Could you check a few things on this model? Use its own coordinates, in mm. A direction names the side the tool comes from. Give positions to 0.01 mm unless a question says otherwise; leave off trailing zeros. Order: outer loops, then holes, each group sorted by start corner. A loop starts at its lowest first (then second) coordinate and runs counter-clockwise, first axis right, second up. Notation, with made-up numbers: (4, 23) - (61, 23) arc R11 ccw to (61, 44) - close; hole circle Ø4 at (57.5, 18.25). An arc over 180 degrees is marked (long way). One line per question, with ' | ' between items. Start each with the question number.
1. Which directions (+Z, -Z, +X, -X, +Y, -Y) give clear straight access to the entire face, cutting with the end or side of a thin tool? Please do faces 5 (the flat face through (1.8, 0, 18)), 6 (the flat face through (1.8, 0, -18)), 7 (the flat face through (1.8, -13, -13)), 8 (the flat face through (6, -14, 0)).
2. Imagine slicing it at A-A (y = 18.5). Please give me the cut outline in (x, z).
3. If we mould it in two halves opening along Z, with no side actions, what happens to faces 1 (the cylindrical face through (2.96, 7.28, -23.13)), 2 (the flat face through (-79, 27.848, 0)), 3 (the cylindrical face through (3.871, 14.888, 13.165)), 4 (the flat face through (1.8, 13, -13))? For each: released by +Z, released by -Z, zero draft, split by the parting line, or undercut.
4. I need wall thicknesses on probe 1 along X at (y, z) = (-10, 2.5); probe 2 along Z at (x, y) = (-78.5, 22.5); probe 3 along X at (y, z) = (17, 12.5). Which ranges of each line are inside material? Lowest first, please. Write a range as from..to.
5. For P1, Ø5, axis at x = -71, z = -6, coming from the -Y side; P2, Ø20.5, axis at y = 6, z = 1.5, coming from the +X side; P3, Ø8, axis at x = 8.5, z = -10.5, coming from the -Y side; P4, Ø4, axis at x = -31.5, y = -18.5, coming from the -Z side, each with a flat end and sliding along its axis, tell me the tip position at first contact or that it passes through.
6. Imagine slicing it at B-B (x = -20.5). Please give me the cut outline in (y, z), and give its area (3 significant figures).
```python
from build123d import *
from build123d.topology import SkipClean

# Parameters (mm, degrees)
SKETCH1_R           = 24.6
BOSS_EXTRUDE1_DEPTH = 87
SKETCH2_R           = 24.25
BOSS_EXTRUDE2_DEPTH = 6
BOSS_EXTRUDE3_DEPTH = 5
CUT_EXTRUDE1_START  = -4.2
SKETCH4_R           = 5.5
SKETCH4_R_2         = 2
CUT_EXTRUDE1_DEPTH  = 4.2
CUT_EXTRUDE2_START  = -0.5
CUT_EXTRUDE2_DEPTH  = 0.5
SKETCH6_R           = 12.7
SKETCH6_R_2         = 5.5
BOSS_EXTRUDE4_DEPTH = 2.5
SKETCH7_R           = 10
SKETCH7_R_2         = 8.5
CUT_EXTRUDE3_DEPTH  = 0.5
SKETCH8_R           = 4
BOSS_EXTRUDE5_DEPTH = 33
CUT_EXTRUDE4_DEPTH  = 3.5
BOSS_EXTRUDE7_START = 22
BOSS_EXTRUDE7_DEPTH = 22


with BuildPart() as part:
    # Sketch1 → Boss-Extrude1 (new body)
    with BuildSketch(Plane(origin=(0, 0, 0), x_dir=(0, 0, -1), z_dir=(1, 0, 0))):
        Circle(SKETCH1_R)
    extrude(amount=-BOSS_EXTRUDE1_DEPTH)

    # Sketch2 → Boss-Extrude2 (add)
    with BuildSketch(Plane(origin=(0, 0, 0), x_dir=(0, 0, -1), z_dir=(1, 0, 0))):
        Circle(SKETCH2_R)
    extrude(amount=BOSS_EXTRUDE2_DEPTH)

    # Sketch3 → Boss-Extrude3 (add)
    with BuildSketch(Plane.ZY.offset(87)):
        with BuildLine():
            Line((11, 27.947721977), (-11, 27.947721977))
            Line((-11, 27.947721977), (-11, 21.947721977))
            ThreePointArc((-11, 21.947721977), (0, -24.55), (11, 21.947721977))
            Line((11, 21.947721977), (11, 27.947721977))
        make_face()
    extrude(amount=BOSS_EXTRUDE3_DEPTH)

    # Sketch4 → Cut-Extrude1 (cut)
    with BuildSketch(Plane(origin=(6, 0, 0), x_dir=(0, 0, -1), z_dir=(1, 0, 0)).offset(CUT_EXTRUDE1_START)):
        Circle(SKETCH4_R)
        with Locations((-12.904698757, 12.904698757)):
            Circle(SKETCH4_R_2)
        with Locations((12.904698757, 12.904698757)):
            Circle(SKETCH4_R_2)
        with Locations((12.904698757, -12.904698757)):
            Circle(SKETCH4_R_2)
        with Locations((-12.904698757, -12.904698757)):
            Circle(SKETCH4_R_2)
        with BuildLine():
            Line((-23.728938029, 5), (-11.674330816, 5))
            ThreePointArc((-11.674330816, 5), (-12.7, 0), (-11.674330816, -5))
            Line((-11.674330816, -5), (-23.728938029, -5))
            ThreePointArc((-23.728938029, -5), (-24.25, 0), (-23.728938029, 5))
        make_face()
        with BuildLine():
            Line((11.674330816, -5), (23.728938029, -5))
            ThreePointArc((23.728938029, -5), (24.25, 0), (23.728938029, 5))
            Line((23.728938029, 5), (11.674330816, 5))
            ThreePointArc((11.674330816, 5), (12.7, 0), (11.674330816, -5))
        make_face()
    extrude(amount=CUT_EXTRUDE1_DEPTH, mode=Mode.SUBTRACT)

    # Sketch5 → Cut-Extrude2 (cut)
    with SkipClean():  # the faces are left unmerged after this step: merging them gives an invalid solid
        with BuildSketch(Plane(origin=(6, 0, 0), x_dir=(0, 0, -1), z_dir=(1, 0, 0)).offset(CUT_EXTRUDE2_START)):
            with BuildLine():
                Line((-11.674330816, 5), (-12.539936204, 5))
                ThreePointArc((-12.539936204, 5), (0, 13.5), (12.539936204, 5))
                Line((12.539936204, 5), (11.674330816, 5))
                ThreePointArc((11.674330816, 5), (0, 12.7), (-11.674330816, 5))
            make_face()
            with BuildLine():
                Line((-11.674330816, -5), (-12.539936204, -5))
                ThreePointArc((-12.539936204, -5), (0, -13.5), (12.539936204, -5))
                Line((12.539936204, -5), (11.674330816, -5))
                ThreePointArc((11.674330816, -5), (0, -12.7), (-11.674330816, -5))
            make_face()
        extrude(amount=CUT_EXTRUDE2_DEPTH, mode=Mode.SUBTRACT)

    # Sketch6 → Boss-Extrude4 (add)
    with BuildSketch(Plane(origin=(6, 0, 0), x_dir=(0, 0, -1), z_dir=(1, 0, 0))):
        Circle(SKETCH6_R)
        Circle(SKETCH6_R_2, mode=Mode.SUBTRACT)
    extrude(amount=BOSS_EXTRUDE4_DEPTH)

    # Sketch7 → Cut-Extrude3 (cut)
    with BuildSketch(Plane(origin=(8.5, 0, 0), x_dir=(0, 0, -1), z_dir=(1, 0, 0))):
        Circle(SKETCH7_R)
        Circle(SKETCH7_R_2, mode=Mode.SUBTRACT)
    extrude(amount=-CUT_EXTRUDE3_DEPTH, mode=Mode.SUBTRACT)

    # Sketch8 → Boss-Extrude5 (add)
    with BuildSketch(Plane(origin=(1.8, 0, 0), x_dir=(0, 0, -1), z_dir=(1, 0, 0))):
        Circle(SKETCH8_R)
    extrude(amount=BOSS_EXTRUDE5_DEPTH)

    # Sketch9 → Cut-Extrude4 (cut)
    with BuildSketch(Plane(origin=(-87, 0, 0), x_dir=(0, 0, -1), z_dir=(1, 0, 0))):
        with BuildLine():
            Line((11, 21.947721977), (11, 27.947721977))
            Line((11, 27.947721977), (-11, 27.947721977))
            Line((-11, 27.947721977), (-11, 21.947721977))
            ThreePointArc((-11, 21.947721977), (0, 24.55), (11, 21.947721977))
        make_face()
    extrude(amount=-CUT_EXTRUDE4_DEPTH, mode=Mode.SUBTRACT)

    # Sketch11 → Boss-Extrude7 (add)
    with BuildSketch(Plane(origin=(-90.5, 0, 0), x_dir=(0, 0, -1), z_dir=(1, 0, 0)).offset(BOSS_EXTRUDE7_START)):
        with BuildLine():
            Line((-9.5, 27.847721977), (-9.5, 23.12466216))
            ThreePointArc((-9.5, 23.12466216), (-10.256840655, 22.799061818), (-11.002541178, 22.448699019))
            Line((-11.002541178, 22.448699019), (-11, 21.947721977))
            ThreePointArc((-11, 21.947721977), (0, 24.55), (11, 21.947721977))
            Line((11, 21.947721977), (11.002541178, 22.448699019))
            ThreePointArc((11.002541178, 22.448699019), (10.256840655, 22.799061818), (9.5, 23.12466216))
            Line((9.5, 23.12466216), (9.5, 27.847721977))
            Line((9.5, 27.847721977), (-9.5, 27.847721977))
        make_face()
    extrude(amount=-BOSS_EXTRUDE7_DEPTH)

    # Sketch12 → Revolve1 (revolve)
    with BuildSketch(Plane.XY, mode=Mode.PRIVATE) as revolve1_sk:
        Polygon((-92, 4), (-97, 4), (-97, 2.5), (-107, 2.5), (-107, 0), (-92, 0), align=None)
    revolve(revolve1_sk.sketch.rotate(Axis((0, 0, 0), (-1, 0, 0)), 90), axis=Axis((0, 0, 0), (-1, 0, 0)))


solid = part.part
```
Results found:
1) face 5: +Z, +X | face 6: -Z, +X | face 7: +X | face 8: +X, -Y
2) outline: (-92, -16.14) - (-87, -16.14) - (-87, -16.21) - (0, -16.21) - (0, -15.68) - (6, -15.68) - (6, 15.68) - (0, 15.68) - (0, 16.21) - (-87, 16.21) - (-87, 16.14) - (-92, 16.14) - close
3) face 1: split by the parting line | face 2: zero draft | face 3: undercut | face 4: undercut
4) probe 1: x = -92..8.5 | probe 2: z = -10.9..10.9 | probe 3: x = -92..6
5) P1: stops at y = -24.35 | P2: stops at x = 34.8 | P3: stops at y = -23.1 | P4: stops at z = -18.25
6) outline: circle Ø49.2 at (0, 0) | area: 1,900 mm2
